Autodesk Inventor part; units mm, degrees
ref_plane "YZ Plane" through (0, 0, 0) normal (1, 0, 0) x (0, 1, 0)
ref_plane "XZ Plane" through (0, 0, 0) normal (0, 1, 0) x (-1, 0, 0)
ref_plane "XY Plane" through (0, 0, 0) normal (0, 0, 1) x (1, 0, 0)
sketch "Sketch9" plane through (0, 0, 0) normal (0, 1, 0) x (-1, 0, 0)
  line L0 (15, 15) -> (-15, 15)
  line L1 (-15, 15) -> (-15, -15)
  line L2 (-15, -15) -> (15, -15)
  line L3 (15, -15) -> (15, 15)
  line L4 (15, 15) -> (-15, -15) construction
  line L5 (-15, 15) -> (15, -15) construction
  line L6 (-13, 13) -> (13, 13)
  line L7 (13, 13) -> (13, -13)
  line L8 (13, -13) -> (-13, -13)
  line L9 (-13, -13) -> (-13, 13)
  point P0 (0, 0)
  dimension "d172" = 30
  dimension "d173" = 30
  dimension "d174" = 2
extrude "Extrusion3" add sketch "Sketch9" against normal blind 515
sketch "Sketch10" plane through (0, 0, 0) normal (1, 0, 0) x (0, 1, 0)
  line L0 (0, 15) -> (0, -15) construction
  line L1 (0, 15) -> (-515, 15) construction
  line L2 (-515, -15) -> (-515, 15) construction
  line L3 (0, -15) -> (-515, -15) construction
  line L4 (-68.5, 8.5) -> (-51.5, 8.5)
  line L5 (-51.5, 8.5) -> (-51.5, -8.5)
  line L6 (-51.5, -8.5) -> (-68.5, -8.5)
  line L7 (-68.5, -8.5) -> (-68.5, 8.5)
  line L8 (-68.5, 8.5) -> (-51.5, -8.5) construction
  line L9 (-51.5, 8.5) -> (-68.5, -8.5) construction
  line L10 (0, 0) -> (30, 0)
  circle A0 centre (-60, 0) radius 8.5
  dimension "d177" = 17
  dimension "d178" = 17
  dimension "d181" = 30
  dimension "d182" = 90
extrude "Extrusion4" cut sketch "Sketch10" along normal through all contours A0
pattern_linear "Rectangular Pattern4" count 4 spacing 85 along (0, -1, 0) of "Extrusion4"
properties part number "PRS 1661 DrSysB way tube 1_1200" material "Stainless Steel"
The model under review builds one solid part; all positions refer to its coordinate system, in mm. A direction names the side the tool comes from. Round coordinates to 2 decimals unless told otherwise and drop trailing zeros. Loops run counter-clockwise (first coordinate to the right, second up) from the corner with the lowest first, then second, coordinate; pieces in that order, holes last. Notation, with made-up numbers: (23.5, 44) - (67.5, 44) arc R24 cw to (67.5, 55) - close; hole circle Ø4 at (67, 35.25). An arc over 180 degrees is marked (long way). Use a Markdown table: item, result. Add a question column.
Q1. Add section B-B (z = 0). State the section outline as (x, y) points.
Q2. Insertion check: pin 1 Ø13.5 at (y, z) = (-145, 0) entering from +X; pin 2 Ø2 at (x, z) = (4, -11.5) entering from -Y. Each pin has a flat end and moves straight along its axis. Give the tip position at first contact, or say it passes through.
Q3. Add section C-C (x = 3.75). State the section outline as (y, z) points.
Q4. Add section A-A (y = -299.5). State the section outline as (x, z) points, plus the area to 3 significant figures.
Q5. The part is to be moulded in two halves that separate along Z. For faces 4 (the face through (13.99, -68.49, -0.37)), 5 (the face through (15, -254, 0)), 6 (the face through (0, -254, -15)), say which applies: pulls with the +Z half, pulls with the -Z half, needs draft (parallel to the pull), parting line crosses it, or undercut.
Q6. Machinability: for faces 1 (the face through (0, -254, -13)), 2 (the face through (14, 0, 0)), 3 (the face through (13.99, -238.49, -0.37)), which of the approach directions +Z, -Z, +X, -X, +Y, -Y give a long, thin tool a straight path to every point of the face, cutting with its end or side? Answer none if there is none.
Q7. For probe 1 along Y at (x, z) = (14.5, 0); probe 2 along Z at (x, y) = (13.9, -60); probe 3 along Z at (x, y) = (9.25, -88.5), list the stretches that pass through material, from the lowest coordinate up.
Worked answers:
| question | item | result |
|---|---|---|
| 1 | outline | (-15, -515) - (-13, -515) - (-13, 0) - (-15, 0) - close; (13, -515) - (15, -515) - (15, -323.5) - (13, -323.5) - close; (13, -306.5) - (15, -306.5) - (15, -238.5) - (13, -238.5) - close; (13, -221.5) - (15, -221.5) - (15, -153.5) - (13, -153.5) - close; (13, -136.5) - (15, -136.5) - (15, -68.5) - (13, -68.5) - close; (13, -51.5) - (15, -51.5) - (15, 0) - (13, 0) - close |
| 2 | pin 1 | x = -13 |
| 2 | pin 2 | through |
| 3 | outline | (-515, -15) - (0, -15) - (0, -13) - (-515, -13) - close; (-515, 13) - (0, 13) - (0, 15) - (-515, 15) - close |
| 4 | outline | (-15, -15) - (15, -15) - (15, 15) - (-15, 15) - close; hole (-13, -13) - (13, -13) - (13, 13) - (-13, 13) - close |
| 4 | area | 224 mm² |
| 5 | face 4 | undercut |
| 5 | face 5 | needs draft |
| 5 | face 6 | pulls with the -Z half |
| 6 | face 1 | +Y, -Y |
| 6 | face 2 | +Z, -Z, +X, -X, +Y |
| 6 | face 3 | +X |
| 7 | probe 1 | -515 to -323.5, -306.5 to -238.5, -221.5 to -153.5, -136.5 to -68.5, -51.5 to 0 |
| 7 | probe 2 | -15 to -8.5, 8.5 to 15 |
| 7 | probe 3 | -15 to -13, 13 to 15 |
